The drawing under review shows one solid part. Ordinate dimensions are in mm from its lowest x, y, z. Round coordinates to 2 decimals unless told otherwise and drop trailing zeros. Order: outer loops, then holes, each group sorted by start corner. A loop starts at its lowest first (then second) coordinate and runs counter-clockwise, first axis right, second up. Notation, with made-up numbers: M 71.25,6.5 L 117.25,6.5 A18 ccw 117.25,39.5 Z; hole C -26,2.5 d5. An arc over 180 degrees is marked long. Answer as a JSON object with one key per item and string values. Group by question number.
1. To check wall thickness, follow probe 1 along Z at (x, y) = (46.5, 1.1) (1 decimal); probe 2 along Z at (x, y) = (27, 0.15). State the ranges of each line that lie inside material, in increasing order. Write a range as [from, to].
2. Add section D-D on x = 26. State the section outline as (y, z) points.
3. Add section B-B on x = 48. State the section outline as (y, z) points (1 decimal).
4. Add section C-C on y = 1.25. State the section outline as (x, z) points (1 decimal).
5. Add section A-A on z = 8. State the section outline as (x, y) points (1 decimal).
6. Clearance check with flat-ended pins moving along their axes: P1, Ø0.5, axis at y = 1, z = 49, coming from the -X side (1 decimal); P2, Ø0.8, axis at x = 47.5, y = 0.5, coming from the +Z side; P3, Ø0.8, axis at y = 1, z = 5.5, coming from the +X side (1 decimal); P4, Ø4, axis at x = 21, z = 28.5, coming from the -Y side. State where each tip first meets the part, or that it passes through.
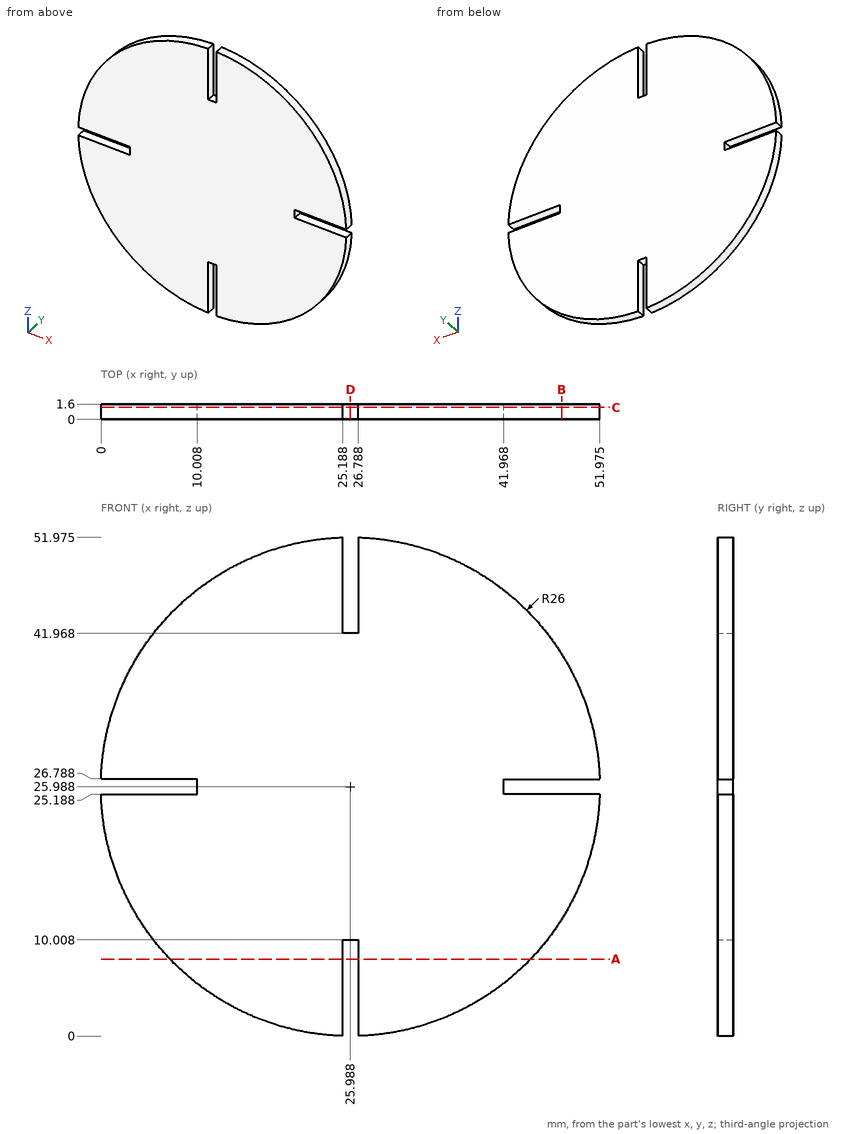
Recorded:
{
 "1": {"probe 1": "z = [10, 25.2], [26.8, 42]", "probe 2": "z = [0.01, 51.97]"},
 "2": {"outline": "M 0,10.01 L 1.6,10.01 L 1.6,41.97 L 0,41.97 Z"},
 "3": {"outline": "M 0,12.2 L 1.6,12.2 L 1.6,25.2 L 0,25.2 Z; M 0,26.8 L 1.6,26.8 L 1.6,39.8 L 0,39.8 Z"},
 "4": {"outline": "M 0,25.2 A26 ccw 25.2,0 L 25.2,10 L 26.8,10 L 26.8,0 A26 ccw 52,25.2 L 42,25.2 L 42,26.8 L 52,26.8 A26 ccw 26.8,52 L 26.8,42 L 25.2,42 L 25.2,52 A26 ccw 0,26.8 L 10,26.8 L 10,25.2 Z"},
 "5": {"outline": "M 7.2,0 L 25.2,0 L 25.2,1.6 L 7.2,1.6 Z; M 26.8,0 L 44.8,0 L 44.8,1.6 L 26.8,1.6 Z"},
 "6": {"P1": "stops at x = 13.4", "P2": "stops at z = 41.16", "P3": "stops at x = 42.5", "P4": "stops at y = 0"}
}
